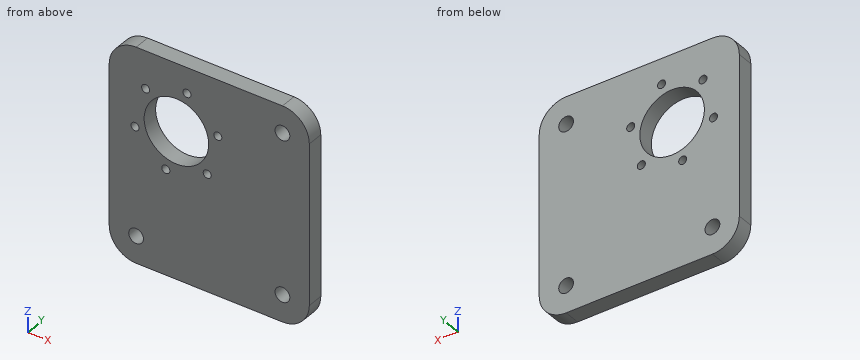
from build123d import *

# Parameters (mm, degrees)
SKETCH2_W           = 74.44
SKETCH2_H           = 79.38
SKETCH2_R           = 12
BOSS_EXTRUDE1_DEPTH = 6
SKETCH6_R           = 2.75
CUT_EXTRUDE2_DEPTH  = 10
SKETCH8_R           = 1.5
CUT_EXTRUDE4_DEPTH  = 7
FILLET1_R           = 10


with BuildPart() as part:
    # Sketch2 → Boss-Extrude1 (new body)
    with BuildSketch(Plane(origin=(0, 0, 0), x_dir=(1, 0, 0), z_dir=(0, 1, 0))):
        with Locations((18.526729133, 13.835644594)):
            Rectangle(SKETCH2_W, SKETCH2_H)
        with Locations((6.306729133, -0.854355406)):
            Circle(SKETCH2_R, mode=Mode.SUBTRACT)
    extrude(amount=BOSS_EXTRUDE1_DEPTH)

    # Sketch6 → Cut-Extrude2 (cut)
    with BuildSketch(Plane.XZ):
        with Locations((45.746729133, 15.854355406)):
            Circle(SKETCH6_R)
        with Locations((45.746729133, -43.525644594)):
            Circle(SKETCH6_R)
        with Locations((-8.693270867, -43.525644594)):
            Circle(SKETCH6_R)
    extrude(amount=-CUT_EXTRUDE2_DEPTH, mode=Mode.SUBTRACT)

    # Sketch8 → Cut-Extrude4 (cut, through all)
    with BuildSketch(Plane.XZ):
        with Locations((21.705664704, 5.198637084)):
            Circle(SKETCH8_R)
        with Locations((17.768455213, -10.30937315)):
            Circle(SKETCH8_R)
        with Locations((2.369519643, -14.653654828)):
            Circle(SKETCH8_R)
        with Locations((-9.092206437, -3.489926272)):
            Circle(SKETCH8_R)
        with Locations((-5.154996946, 12.018083962)):
            Circle(SKETCH8_R)
        with Locations((10.243938624, 16.36236564)):
            Circle(SKETCH8_R)
    extrude(amount=-CUT_EXTRUDE4_DEPTH, mode=Mode.SUBTRACT)

    # Fillet1
    fillet1_edges = [part.edges().sort_by_distance(p)[0] for p in [
        (-18.693270867, 3, -53.525644594),
        (55.746729133, 3, -53.525644594),
        (55.746729133, 3, 25.854355406),
        (-18.693270867, 3, 25.854355406),
    ]]
    fillet(fillet1_edges, radius=FILLET1_R)


solid = part.part
Verification items for the finished model (mm, model axes). Round coordinates to 2 decimals unless told otherwise and drop trailing zeros. Loops run counter-clockwise (first coordinate to the right, second up) from the corner with the lowest first, then second, coordinate; pieces in that order, holes last. Notation, with made-up numbers: (-13.75, 41) - (43.25, 41) arc R13 cw to (43.25, 54) - close; hole circle Ø4 at (88.25, 35.5). An arc over 180 degrees is marked (long way). Use a Markdown table: item, result. Add a question column.
1. Gauge pin test, flat end, axial feed: pin 1 (6 mm diameter, centred on x = 15, z = -5.5, fed in from +Y). Record the tip position at first contact, or that the pin passes through.
2. Section check B-B, the plane z = -7.5. Record the boundary of the cut face in (x, y), plus the area to 3 significant figures.
3. Section check D-D, the plane z = 2.5. Record the boundary of the cut face in (x, y), plus the area to 3 significant figures.
4. Section check A-A, the plane x = 10.5. Record the boundary of the cut face in (y, z).
5. Thickness scan on probe 1 along X at (y, z) = (3.45, 4); probe 2 along X at (y, z) = (4.8, 17); probe 3 along Z at (x, y) = (10, 4.4). Record the ranges inside material, lowest first. Write a range as [from, to].
6. Section check C-C, the plane y = 1. Give the number of separate pieces and of enclosed holes in the cut face, plus the area to 3 significant figures.
Checks:
| question | item | result |
|---|---|---|
| 1 | pin 1 | stops at y = 6 |
| 2 | outline | (-18.69, 0) - (-2.31, 0) - (-2.31, 6) - (-18.69, 6) - close; (14.92, 0) - (55.75, 0) - (55.75, 6) - (14.92, 6) - close |
| 2 | area | 343 mm^2 |
| 3 | outline | (-18.69, 0) - (-5.58, 0) - (-5.58, 6) - (-18.69, 6) - close; (18.19, 0) - (55.75, 0) - (55.75, 6) - (18.19, 6) - close |
| 3 | area | 304 mm^2 |
| 4 | outline | (0, -53.53) - (6, -53.53) - (6, -10.39) - (0, -10.39) - close; (0, 12.1) - (6, 12.1) - (6, 14.88) - (0, 14.88) - close; (0, 17.84) - (6, 17.84) - (6, 25.85) - (0, 25.85) - close |
| 5 | probe 1 | x = [-18.69, -5.27], [17.89, 20.8], [22.61, 55.75] |
| 5 | probe 2 | x = [-18.63, 8.89], [11.6, 43.25], [48.25, 55.68] |
| 5 | probe 3 | z = [-53.53, -10.56], [12.27, 14.88], [17.84, 25.85] |
| 6 | separate pieces | 1 |
| 6 | enclosed holes | 10 |
| 6 | area | 5,260 mm^2 |
